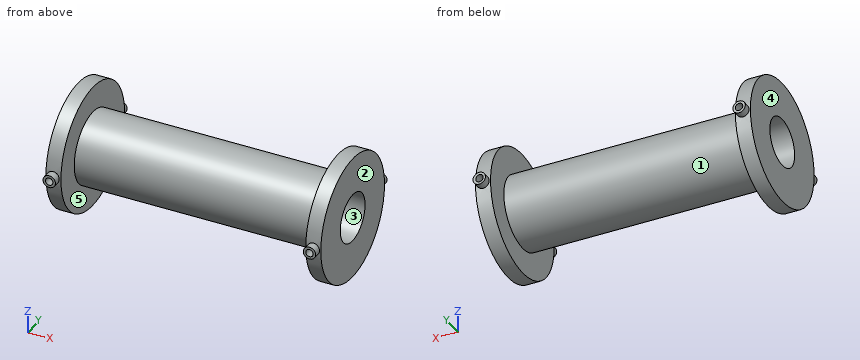
```python
from build123d import *

# Parameters (mm, degrees)
CROQUIS3_R              = 5
SALIENTE_EXTRUIR1_DEPTH = 6
CROQUIS4_R              = 3
CORTAR_EXTRUIR1_DEPTH   = 12
CROQUIS5_R              = 5
SALIENTE_EXTRUIR2_DEPTH = 6
CROQUIS6_R              = 3
CORTAR_EXTRUIR2_DEPTH   = 12
CROQUIS8_R              = 5
SALIENTE_EXTRUIR4_DEPTH = 6
CROQUIS9_R              = 3
CORTAR_EXTRUIR4_DEPTH   = 12
CROQUIS10_R             = 5
SALIENTE_EXTRUIR5_DEPTH = 6
CROQUIS11_R             = 3
CORTAR_EXTRUIR5_DEPTH   = 12


with BuildPart() as part:
    # Camisa → Revolución3 (revolve)
    with BuildSketch(Plane.XY):
        Polygon((-110.61, 19.5), (110.61, 19.5), (110.61, 50.1), (98.51, 50.1), (98.51, 29.193885615), (-98.51, 29.193885615), (-98.51, 50.1), (-110.61, 50.1), align=None)
        Polygon((100.51, 48.1), (108.61, 48.1), (108.61, 21.5), (-108.61, 21.5), (-108.61, 48.1), (-100.51, 48.1), (-100.51, 27.193885615), (100.51, 27.193885615), align=None, mode=Mode.SUBTRACT)
    revolve(axis=Axis((125, 0, 0), (-1, 0, 0)))

    # Croquis3 → Saliente-Extruir1 (add, symmetric)
    with BuildSketch(Plane(origin=(0, 50.1, 0), x_dir=(1, 0, 0), z_dir=(0, 1, 0))):
        with Locations(Location((-104.56, 0, 0), (0, 0, 180))):
            Circle(CROQUIS3_R)
    extrude(amount=SALIENTE_EXTRUIR1_DEPTH, both=True)

    # Croquis4 → Cortar-Extruir1 (cut)
    with BuildSketch(Plane(origin=(0, 56.1, 0), x_dir=(1, 0, 0), z_dir=(0, 1, 0))):
        with Locations(Location((-104.56, 0, 0), (0, 0, 180))):
            Circle(CROQUIS4_R)
    extrude(amount=-CORTAR_EXTRUIR1_DEPTH, mode=Mode.SUBTRACT)

    # Croquis5 → Saliente-Extruir2 (add, symmetric)
    with BuildSketch(Plane(origin=(0, 50.1, 0), x_dir=(1, 0, 0), z_dir=(0, 1, 0))):
        with Locations(Location((104.56, 0, 0), (0, 0, 180))):
            Circle(CROQUIS5_R)
    extrude(amount=SALIENTE_EXTRUIR2_DEPTH, both=True)

    # Croquis6 → Cortar-Extruir2 (cut)
    with BuildSketch(Plane(origin=(0, 56.1, 0), x_dir=(1, 0, 0), z_dir=(0, 1, 0))):
        with Locations(Location((104.311648401, 0, 0), (0, 0, 180))):
            Circle(CROQUIS6_R)
    extrude(amount=-CORTAR_EXTRUIR2_DEPTH, mode=Mode.SUBTRACT)

    # Croquis8 → Saliente-Extruir4 (add, symmetric)
    with BuildSketch(Plane(origin=(0, -50.1, 0), x_dir=(-1, 0, 0), z_dir=(0, -1, 0))):
        with Locations((104.879923699, 0)):
            Circle(CROQUIS8_R)
    extrude(amount=SALIENTE_EXTRUIR4_DEPTH, both=True)

    # Croquis9 → Cortar-Extruir4 (cut)
    with BuildSketch(Plane.XZ.offset(56.1)):
        with Locations((-104.879923699, 0)):
            Circle(CROQUIS9_R)
    extrude(amount=-CORTAR_EXTRUIR4_DEPTH, mode=Mode.SUBTRACT)

    # Croquis10 → Saliente-Extruir5 (add, symmetric)
    with BuildSketch(Plane(origin=(0, -50.1, 0), x_dir=(-1, 0, 0), z_dir=(0, -1, 0))):
        with Locations((-104.56, 0)):
            Circle(CROQUIS10_R)
    extrude(amount=SALIENTE_EXTRUIR5_DEPTH, both=True)

    # Croquis11 → Cortar-Extruir5 (cut)
    with BuildSketch(Plane.XZ.offset(56.1)):
        with Locations((104.56, 0)):
            Circle(CROQUIS11_R)
    extrude(amount=-CORTAR_EXTRUIR5_DEPTH, mode=Mode.SUBTRACT)


solid = part.part
```
For this review, take the finished solid that the model builds, in its own axes (mm). Face numbers are marked on the shaded views. A direction names the side the tool comes from. Round coordinates to 2 decimals unless told otherwise and drop trailing zeros. Loops run counter-clockwise (first coordinate to the right, second up) from the corner with the lowest first, then second, coordinate; pieces in that order, holes last.
(1) Wall thickness on line 1 along Y through (x, z) = (-56, 0); line 2 along X through (y, z) = (-1, -34.5): over which ranges is each line inside the solid? List them lowest first.
Returned:
line 1: y = -29.19 to -27.19, -21.5 to -19.5, 19.5 to 21.5, 27.19 to 29.19
line 2: x = -110.61 to -108.61, -100.51 to -98.51, 98.51 to 100.51, 108.61 to 110.61
(2) Tool access review of the marked faces 4 and 5: name each direction out of +Z, -Z, +X, -X, +Y, -Y from which nothing blocks a thin tool from reaching the whole face with its end or side.
Returned:
face 4: +Z, -Z, -X, +Y, -Y
face 5: none
(3) We need section D-D (x = -52). Give the boundary of the cut face in (y, z).
Returned:
outline: circle Ø58.39 at (0, 0); circle Ø43 at (0, 0); hole circle Ø54.39 at (0, 0); hole circle Ø39 at (0, 0)
(4) Clearance check with flat-ended pins moving along their axes: P1, Ø9.5, axis at x = -104.88, z = 0, coming from the +Y side; P2, Ø6, axis at x = 72.5, y = 22, coming from the -Z side; P3, Ø5, axis at x = 104.31, z = 0, coming from the -Y side; P4, Ø1.5, axis at x = 70, y = 22, coming from the -Z side. State where each tip first meets the part, or that it passes through.
Returned:
P1: stops at y = 56.1
P2: stops at z = -22.16
P3: stops at y = -21.5
P4: stops at z = -20.02
(5) Mouldability with a two-part tool opening along Z and no side actions: class the marked faces 1, 2 and 3 as released by +Z, released by -Z, zero draft, split by the parting line, or undercut.
Returned:
face 1: split by the parting line
face 2: zero draft
face 3: undercut
(6) We need section B-B (x = -104.56). Give the boundary of the cut face in (y, z).
Returned:
outline: (-56.1, -4.99) - (-49.85, -4.99) arc R50.1 ccw to (49.85, -5) - (56.1, -5) - (56.1, -3) - (44.1, -3) - (44.1, -5) - (47.84, -5) arc R48.1 cw to (-47.84, -4.99) - (-44.1, -4.99) - (-44.1, -2.98) - (-56.1, -2.98) - close; (-56.1, 2.98) - (-44.1, 2.98) - (-44.1, 4.99) - (-47.84, 4.99) arc R48.1 cw to (47.84, 5) - (44.1, 5) - (44.1, 3) - (56.1, 3) - (56.1, 5) - (49.85, 5) arc R50.1 ccw to (-49.85, 4.99) - (-56.1, 4.99) - close; circle Ø43 at (0, 0); hole circle Ø39 at (0, 0)
(7) We need section C-C (y = 11). State how many separate pieces and enclosed holes the cut face has, plus the area to 3 significant figures.
Returned:
separate pieces: 2
enclosed holes: 2
area: 2,410 mm2
(8) We need section A-A (z = -42.5). Give the boundary of the cut face in (x, y), plus the area to 3 significant figures.
Returned:
outline: (-110.61, -26.53) - (-98.51, -26.53) - (-98.51, 26.53) - (-110.61, 26.53) - close; (98.51, -26.53) - (110.61, -26.53) - (110.61, 26.53) - (98.51, 26.53) - close; hole (-108.61, -22.52) - (-100.51, -22.52) - (-100.51, 22.52) - (-108.61, 22.52) - close; hole (100.51, -22.52) - (108.61, -22.52) - (108.61, 22.52) - (100.51, 22.52) - close
area: 554 mm2
